The model under review builds one solid part; all positions refer to its coordinate system, in mm. Face numbers are marked on the shaded views. A direction names the side the tool comes from. Round coordinates to 2 decimals unless told otherwise and drop trailing zeros. Order: outer loops, then holes, each group sorted by start corner. A loop starts at its lowest first (then second) coordinate and runs counter-clockwise, first axis right, second up. Notation, with made-up numbers: M 23.5,-36 L 48.5,-36 A20 cw 48.5,0 Z; hole C 77,15 d5. An arc over 180 degrees is marked long. One line per item, written item: value. Start each with the question number.
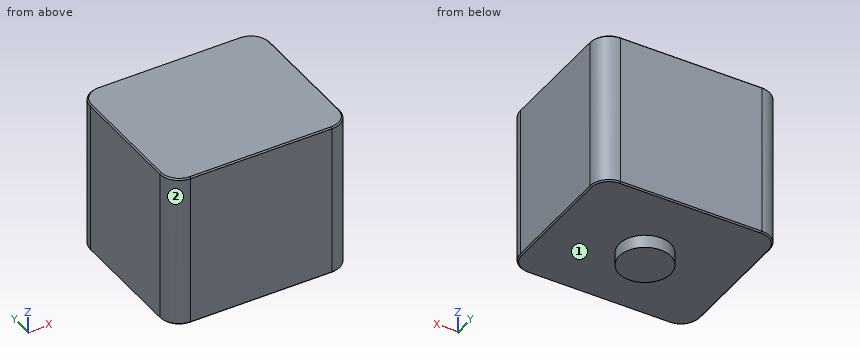
from build123d import *

# Parameters (mm, degrees)
F1_DEPTH = 12
F2_SIZE  = 0.1
F3_R     = 2
F4_DEPTH = 1


with BuildPart() as f1:
    # F0 (on Top) → F1 (new body)
    with BuildSketch(Plane.XY):
        with BuildLine():
            Line((-5.5, -6), (5.5, -6))
            ThreePointArc((5.5, -6), (6.56066, -5.56066), (7, -4.5))
            Line((7, -4.5), (7, 4.5))
            ThreePointArc((7, 4.5), (6.56066, 5.56066), (5.5, 6))
            Line((5.5, 6), (-5.5, 6))
            ThreePointArc((-5.5, 6), (-6.56066, 5.56066), (-7, 4.5))
            Line((-7, 4.5), (-7, -4.5))
            ThreePointArc((-7, -4.5), (-6.56066, -5.56066), (-5.5, -6))
        make_face()
    extrude(amount=F1_DEPTH)

    # F2
    f2_edges = [f1.edges().sort_by_distance(p)[0] for p in [
        (0, -6, 12),
        (6.56066, -5.56066, 12),
        (7, 0, 12),
        (6.56066, 5.56066, 12),
        (0, 6, 12),
        (-6.56066, 5.56066, 12),
        (-7, 0, 12),
        (-6.56066, -5.56066, 12),
        (0, -6, 0),
        (6.56066, -5.56066, 0),
        (7, 0, 0),
        (6.56066, 5.56066, 0),
        (0, 6, 0),
        (-6.56066, 5.56066, 0),
        (-7, 0, 0),
        (-6.56066, -5.56066, 0),
    ]]
    chamfer(f2_edges, length=F2_SIZE)

    # F3 (on face) → F4 (join)
    with BuildSketch(Plane(origin=(0, 0, 0), x_dir=(1, 0, 0), z_dir=(0, 0, -1))):
        Circle(F3_R)
    extrude(amount=F4_DEPTH)


solid = f1.part
Item 1: Consider section D-D, the plane x = 4.75. Give the boundary of the cut face in (y, z), then the cut area to 3 significant figures.
Item 2: Machinability: for the marked faces 1 and 2, which of the approach directions +Z, -Z, +X, -X, +Y, -Y give a long, thin tool a straight path to every point of the face, cutting with its end or side? Answer none if there is none.
Item 3: Consider section C-C, the plane y = 0. Give the boundary of the cut face in (x, z), then the cut area to 3 significant figures.
Item 4: Consider section B-B, the plane y = 2.25. Give the boundary of the cut face in (x, z), then the cut area to 3 significant figures.
Item 5: Wall thickness on L1, parallel to Z at x = -5.25, y = 4.5; L2, parallel to Y at x = -6.25, z = 11; L3, parallel to Y at x = -6, z = 11.25: over which ranges is each line inside the solid? List them lowest first.
Item 6: Consider section A-A, the plane x = 0. Give the boundary of the cut face in (y, z).
Computed:
1. outline: M -6,0.1 L -5.9,0 L 5.9,0 L 6,0.1 L 6,11.9 L 5.9,12 L -5.9,12 L -6,11.9 Z
1. area: 144 mm^2
2. face 1: -Z
2. face 2: +Z, -Z, -X, -Y
3. outline: M -7,0.1 L -6.9,0 L -2,0 L -2,-1 L 2,-1 L 2,0 L 6.9,0 L 7,0.1 L 7,11.9 L 6.9,12 L -6.9,12 L -7,11.9 Z
3. area: 172 mm^2
4. outline: M -7,0.1 L -6.9,0 L 6.9,0 L 7,0.1 L 7,11.9 L 6.9,12 L -6.9,12 L -7,11.9 Z
4. area: 168 mm^2
5. L1: z = 0 to 12
5. L2: y = -5.8 to 5.8
5. L3: y = -5.91 to 5.91
6. outline: M -6,0.1 L -5.9,0 L -2,0 L -2,-1 L 2,-1 L 2,0 L 5.9,0 L 6,0.1 L 6,11.9 L 5.9,12 L -5.9,12 L -6,11.9 Z
